from build123d import *

# Parameters (mm, degrees)
SKETCH1_W                = 56.4
SKETCH1_H                = 56.4
BOSS_EXTRUDE1_DEPTH      = 5
SKETCH2_R                = 19.05
BOSS_EXTRUDE2_DEPTH      = 1.6
SKETCH3_R                = 4
SHALF_DEPTH              = 23.4
CHAMFER1_SIZE            = 0.5
CUT_EXTRUDE1_DEPTH       = 48.068885689
CUT_EXTRUDE1_DEPTH_BACK  = 48.068885689
SKETCH4_R                = 2.6
FILLET1_R                = 3
BOSS_EXTRUDE4_DEPTH      = 46
FILLET2_R                = 3
BOSS_EXTRUDE5_DEPTH      = 5.5
BOSS_EXTRUDE5_DEPTH_BACK = 5
SKETCH6_W                = 7
SKETCH6_H                = 32.2


with BuildPart() as part:
    # Sketch1 → Boss-Extrude1 (new body)
    with BuildSketch(Plane.XY):
        Rectangle(SKETCH1_W, SKETCH1_H)
    extrude(amount=-BOSS_EXTRUDE1_DEPTH)

    # Sketch2 → Boss-Extrude2 (add)
    with BuildSketch(Plane.XY):
        Circle(SKETCH2_R)
    extrude(amount=BOSS_EXTRUDE2_DEPTH)

    # Sketch3 → Shalf (add)
    with BuildSketch(Plane.XY.offset(1.6)):
        Circle(SKETCH3_R)
    extrude(amount=SHALF_DEPTH)

    # Chamfer1
    chamfer1_edges = [part.edges().sort_by_distance(p)[0] for p in [
        (-4, 0, 25),
    ]]
    chamfer(chamfer1_edges, length=CHAMFER1_SIZE)

    # Sketch4 → Cut-Extrude1 (cut, two sides: drawn at the far end of the back side and taken through both)
    with BuildSketch(Plane.XY.offset(-CUT_EXTRUDE1_DEPTH_BACK)):
        with Locations((-23.57, 23.57)):
            Circle(SKETCH4_R)
        with Locations((23.57, 23.57)):
            Circle(SKETCH4_R)
        with Locations((-23.57, -23.57)):
            Circle(SKETCH4_R)
        with Locations((23.57, -23.57)):
            Circle(SKETCH4_R)
    extrude(amount=CUT_EXTRUDE1_DEPTH + CUT_EXTRUDE1_DEPTH_BACK, mode=Mode.SUBTRACT)

    # Fillet1
    fillet1_edges = [part.edges().sort_by_distance(p)[0] for p in [
        (28.2, -28.2, -2.5),
        (-28.2, -28.2, -2.5),
        (-28.2, 28.2, -2.5),
        (28.2, 28.2, -2.5),
    ]]
    fillet(fillet1_edges, radius=FILLET1_R)

    # Sketch5 → Boss-Extrude4 (add)
    with BuildSketch(Plane(origin=(0, 0, -5), x_dir=(-1, 0, 0), z_dir=(0, 0, -1))):
        Polygon((-18.2, 28.2), (18.2, 28.2), (18.2, 18.2), (28.2, 18.2), (28.2, -18.2), (18.2, -18.2), (18.2, -28.2), (-18.2, -28.2), (-18.2, -18.2), (-28.2, -18.2), (-28.2, 18.2), (-18.2, 18.2), align=None)
    extrude(amount=BOSS_EXTRUDE4_DEPTH)

    # Fillet2
    fillet2_edges = [part.edges().sort_by_distance(p)[0] for p in [
        (-18.2, 18.2, -28),
        (-18.2, 28.2, -28),
        (18.2, 28.2, -28),
        (18.2, 18.2, -28),
        (28.2, 18.2, -28),
        (28.2, -18.2, -28),
        (18.2, -18.2, -28),
        (18.2, -28.2, -28),
        (-18.2, -28.2, -28),
        (-18.2, -18.2, -28),
        (-28.2, -18.2, -28),
        (-28.2, 18.2, -28),
    ]]
    fillet(fillet2_edges, radius=FILLET2_R)

    # Sketch6 → Boss-Extrude5 (add, two sides: drawn at the far end of the back side and taken through both)
    with BuildSketch(Plane(origin=(28.2, 0, 0), x_dir=(0, 0, -1), z_dir=(1, 0, 0)).offset(-BOSS_EXTRUDE5_DEPTH_BACK)):
        with Locations((45.5, 0)):
            Rectangle(SKETCH6_W, SKETCH6_H)
    extrude(amount=BOSS_EXTRUDE5_DEPTH + BOSS_EXTRUDE5_DEPTH_BACK)


solid = part.part
The model under review builds one solid part; all positions refer to its coordinate system, in mm. A direction names the side the tool comes from. Round coordinates to 2 decimals unless told otherwise and drop trailing zeros. Order: outer loops, then holes, each group sorted by start corner. A loop starts at its lowest first (then second) coordinate and runs counter-clockwise, first axis right, second up. Notation, with made-up numbers: (83.5, 88.5) -> (110.5, 88.5) arc R18 cw to (110.5, 103.5) -> close; hole circle Ø8 at (25.25, 68.5). An arc over 180 degrees is marked (long way). Return JSON: item names as keys, results as strings.
1. Take a section at C-C (z = -24). Write out the cut boundary in (x, y).
Answer block:
{"outline": "(-28.2, -15.2) arc R3 ccw to (-25.2, -18.2) -> (-21.2, -18.2) arc R3 cw to (-18.2, -21.2) -> (-18.2, -25.2) arc R3 ccw to (-15.2, -28.2) -> (15.2, -28.2) arc R3 ccw to (18.2, -25.2) -> (18.2, -21.2) arc R3 cw to (21.2, -18.2) -> (25.2, -18.2) arc R3 ccw to (28.2, -15.2) -> (28.2, 15.2) arc R3 ccw to (25.2, 18.2) -> (21.2, 18.2) arc R3 cw to (18.2, 21.2) -> (18.2, 25.2) arc R3 ccw to (15.2, 28.2) -> (-15.2, 28.2) arc R3 ccw to (-18.2, 25.2) -> (-18.2, 21.2) arc R3 cw to (-21.2, 18.2) -> (-25.2, 18.2) arc R3 ccw to (-28.2, 15.2) -> close"}
2. The part is to be moulded in two halves that separate along X. For faces 1 (the face through (31, -16.1, -45)), 2 (the face through (19.06, 19.1, -28.32)), 3 (the face through (20.973, 23.684, -2.535)), 4 (the face through (-27.34, -27.3, -2.54)), say which applies: +X half, -X half, draft (parallel to the pull), parting line (faces both ways), or undercut.
Answer block:
{"face 1": "draft", "face 2": "+X half", "face 3": "undercut", "face 4": "-X half"}
3. Take a section at A-A (x = 23.57). Write out the cut boundary in (y, z), then the cut area to 3 significant figures.
Answer block:
{"outline": "(-28.2, -5) -> (-26.17, -5) -> (-26.17, 0) -> (-28.2, 0) -> close; (-20.97, -5) -> (-18.2, -5) -> (-18.2, -51) -> (18.2, -51) -> (18.2, -5) -> (20.97, -5) -> (20.97, 0) -> (-20.97, 0) -> close; (26.17, -5) -> (28.2, -5) -> (28.2, 0) -> (26.17, 0) -> close", "area": "1,900 mm²"}
4. For faces 5 (the face through (-18.2, 23, -28)), 6 (the face through (28.2, 0, -50)), 7 (the face through (18.2, -23, -28)), list the 3-axis set-ups (+Z, -Z, +X, -X, +Y, -Y) from which the entire face can be reached by the end or side of a thin tool; tool diameter is ignored.
Answer block:
{"face 5": "-Z, -X, +Y", "face 6": "-Z, +X, +Y, -Y", "face 7": "-Z, +X, -Y"}
5. For L1, parallel to Y at x = -23.57, z = -1.9; L2, parallel to X at y = 23, z = -1, list the stretches that pass through material, from the lowest coordinate up. Write a range as [from, to].
Answer block:
{"L1": "y = [-28.2, -26.17], [-20.97, 20.97], [26.17, 28.2]", "L2": "x = [-28.2, -26.11], [-21.03, 21.03], [26.11, 28.2]"}
6. Take a section at D-D (x = 0). Write out the cut boundary in (y, z), then the cut area to 3 significant figures.
Answer block:
{"outline": "(-28.2, -51) -> (28.2, -51) -> (28.2, 0) -> (19.05, 0) -> (19.05, 1.6) -> (4, 1.6) -> (4, 24.5) -> (3.5, 25) -> (-3.5, 25) -> (-4, 24.5) -> (-4, 1.6) -> (-19.05, 1.6) -> (-19.05, 0) -> (-28.2, 0) -> close", "area": "3,120 mm²"}
7. Insertion check: P1, Ø3, axis at x = -23.57, y = -23.57, coming from the -Z side; P2, Ø3, axis at x = 31.5, z = -46, coming from the -Y side; P3, Ø1.2, axis at y = -24, z = -20, coming from the +X side; P4, Ø3, axis at x = -24, z = -21.5, coming from the -Y side. Each pin has a flat end and moves straight along its axis. Give the tip position at first contact, or say it passes through.
Answer block:
{"P1": "passes through", "P2": "stops at y = -16.1", "P3": "stops at x = 18.2", "P4": "stops at y = -18.2"}
